Work out the finished part from the listing and answer in its coordinate system (mm). Face numbers are marked on the shaded views. A direction names the side the tool comes from. Give positions to 0.01 mm unless a question says otherwise; leave off trailing zeros. Write each loop counter-clockwise with the first axis right and the second up, starting at its lowest first coordinate (ties: lowest second). Pieces come first, ordered by that corner, then holes.
1) Straight lines are drawn through the part: probe 1 along Z at (x, y) = (66, -5.5); probe 2 along Z at (x, y) = (387.5, 24); probe 3 along X at (y, z) = (99, 5.5). For each, find the intervals that lie inside material, in ascending order.
2) Find section C-C (x = 113.5). Determine the outline of the cut face in (y, z), plus the area to 3 significant figures.
3) Find section D-D (y = 95). Determine the outline of the cut face in (x, z), plus the area to 3 significant figures.
4) A tool of negligible diameter and unlimited length cuts with its end or side. For the marked faces 1, 2, 3 and 4, from which of +Z, -Z, +X, -X, +Y, -Y can it reach the whole face along a straight path? Write none if from no direction.
5) Find section A-A (y = 47). Determine the outline of the cut face in (x, z), plus the area to 3 significant figures.
6) Find section B-B (z = 27). Determine the outline of the cut face in (x, y).
7) Given pin 1 Ø18.5 at (x, z) = (21, 29.5) entering from +Y; pin 2 Ø0.9 at (x, y) = (101, -7) entering from +Z; pin 3 Ø12 at (x, y) = (280.78, 11.55) entering from +Z; pin 4 Ø1 at (y, z) = (24.5, 27.5) entering from +X, each flat-ended and moving along its own axis, determine where each tip first touches the part or whether it passes through.
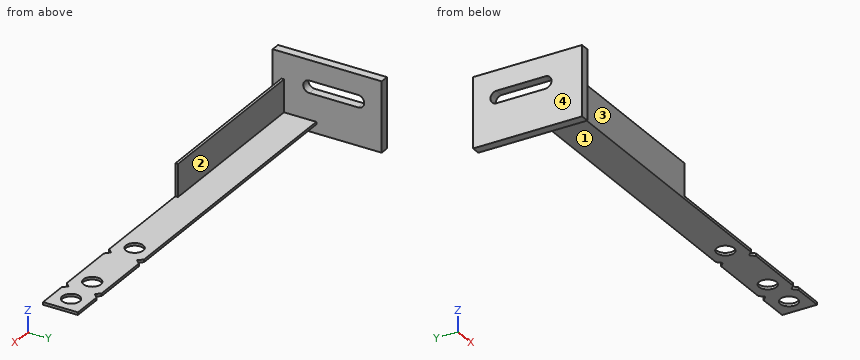
```python
from build123d import *

# Parameters (mm, degrees)
F1_DEPTH = 80
F2_START = 10
F0_R     = 10
F2_DEPTH = 3
F3_START = 10
F3_DEPTH = 40
F5_DEPTH = 25


with BuildPart() as f1:
    # F0 (on Top) → F1 (new body)
    with BuildSketch(Plane.XY):
        Polygon((-39.2155684531, 106.5547373146), (-39.2155684531, -18.4452626854), (-29.2155684531, -18.4452626854), (-29.2155684531, -8.4452626854), (-29.2155684531, -5.4452626854), (-29.2155684531, 31.5547373146), (-29.2155684531, 106.5547373146), align=None)
    extrude(amount=F1_DEPTH)

    # F0 (on Top) → F2 (join)
    with BuildSketch(Plane.XY.offset(F2_START)):
        Polygon((-29.2155684531, 31.5547373146), (-29.2155684531, -5.4452626854), (170.7844315469, -5.4452626854), (170.7844315469, -8.4452626854), (295.7844315469, -8.4452626854), (300.7844315469, -3.4452626854), (305.7844315469, -8.4452626854), (375.7844315469, -8.4452626854), (380.7844315469, -3.4452626854), (385.7844315469, -8.4452626854), (420.7844315469, -8.4452626854), (420.7844315469, 31.5547373146), (385.7844315469, 31.5547373146), (380.7844315469, 26.5547373146), (375.7844315469, 31.5547373146), (305.7844315469, 31.5547373146), (300.7844315469, 26.5547373146), (295.7844315469, 31.5547373146), align=None)
        with Locations((280.7844315469, 11.5547373146)):
            Circle(F0_R, mode=Mode.SUBTRACT)
        with Locations((360.7844315469, 11.5547373146)):
            Circle(F0_R, mode=Mode.SUBTRACT)
        with Locations((400.7844315469, 11.5547373146)):
            Circle(F0_R, mode=Mode.SUBTRACT)
    extrude(amount=F2_DEPTH)

    # F0 (on Top) → F3 (join)
    with BuildSketch(Plane.XY.offset(F3_START)):
        Polygon((-29.2155684531, -5.4452626854), (-29.2155684531, -8.4452626854), (-19.2155684531, -8.4452626854), (170.7844315469, -8.4452626854), (170.7844315469, -5.4452626854), align=None)
    extrude(amount=F3_DEPTH)

    # F4 (on face) → F5 (cut)
    with BuildSketch(Plane.YZ.offset(-29.2155684531)):
        with BuildLine():
            ThreePointArc((23.5547373146, 57), (28.5044847829, 54.9497474683), (30.5547373146, 50))
            ThreePointArc((30.5547373146, 50), (28.5044847829, 45.0502525317), (23.5547373146, 43))
            Line((23.5547373146, 43), (79.5547373146, 43))
            ThreePointArc((79.5547373146, 43), (72.5547373146, 50), (79.5547373146, 57))
            Line((79.5547373146, 57), (23.5547373146, 57))
        make_face()
        with BuildLine():
            ThreePointArc((23.5547373146, 43), (28.5044847829, 45.0502525317), (30.5547373146, 50))
            ThreePointArc((30.5547373146, 50), (28.5044847829, 54.9497474683), (23.5547373146, 57))
            ThreePointArc((23.5547373146, 57), (16.5547373146, 50), (23.5547373146, 43))
        make_face()
        with BuildLine():
            ThreePointArc((86.5547373146, 50), (84.5044847829, 54.9497474683), (79.5547373146, 57))
            ThreePointArc((79.5547373146, 57), (72.5547373146, 50), (79.5547373146, 43))
            ThreePointArc((79.5547373146, 43), (84.5044847829, 45.0502525317), (86.5547373146, 50))
        make_face()
    extrude(amount=-F5_DEPTH, mode=Mode.SUBTRACT)


solid = f1.part
```
Results:
1. probe 1: z = 10 to 50
1. probe 2: z = 10 to 13
1. probe 3: x = -39.22 to -29.22
2. outline: (-8.45, 10) - (31.55, 10) - (31.55, 13) - (-5.45, 13) - (-5.45, 50) - (-8.45, 50) - close
2. area: 231 mm2
3. outline: (-39.22, 0) - (-29.22, 0) - (-29.22, 80) - (-39.22, 80) - close
3. area: 800 mm2
4. face 1: -Z, +X, +Y, -Y
4. face 2: +Z, +X, +Y
4. face 3: +Z, -Z, +X, -Y
4. face 4: +Z, -Z, -X, +Y, -Y
5. outline: (-39.22, 0) - (-29.22, 0) - (-29.22, 43) - (-39.22, 43) - close; (-39.22, 57) - (-29.22, 57) - (-29.22, 80) - (-39.22, 80) - close
5. area: 660 mm2
6. outline: (-39.22, -18.45) - (-29.22, -18.45) - (-29.22, -8.45) - (170.78, -8.45) - (170.78, -5.45) - (-29.22, -5.45) - (-29.22, 106.55) - (-39.22, 106.55) - close
7. pin 1: stops at y = -5.45
7. pin 2: stops at z = 50
7. pin 3: passes through
7. pin 4: stops at x = -29.22
